Part model, mm, in its own coordinate system. A direction names the side the tool comes from. Coordinates: 2 decimals unless noted, no trailing zeros. Loops run counter-clockwise (first coordinate to the right, second up) from the corner with the lowest first, then second, coordinate; pieces in that order, holes last. Notation, with made-up numbers: (57.25, 63) -> (102.25, 63) arc R26 cw to (102.25, 92) -> close; hole circle Ø9 at (2, 33). An arc over 180 degrees is marked (long way). Use one line per item in the form item = value. Start each with the question number.
(1) Band-saw the part on D-D on y = 14.25. Give the cut face in (x, z), then the cut area to 3 significant figures.
(2) Band-saw the part on C-C on y = 8.5. Give the cut face in (x, z).
(3) Band-saw the part on B-B on x = 0. Give the cut face in (y, z), then the cut area to 3 significant figures.
(4) Drill centre lines: L1, parallel to Z at x = 0, y = 1.9; L2, parallel to Y at x = 0.5, z = -0.5; L3, parallel to Y at x = -2.75, z = -4.25. Where is each one in solid material? Low to high. Write a range as [from, to].
(5) Band-saw the part on A-A on z = 0. Give the cut face in (x, y), then the cut area to 3 significant figures.
(6) Pin check, flat tips, straight feed: P1, Ø1, axis at x = -2.5, y = 8, coming from the -Z side; P2, Ø1.5, axis at y = 3, z = 3.5, coming from the +X side; P3, Ø1.5, axis at x = 3.5, y = 10.5, coming from the -Z side. Stop position of each tip, or through.
(7) 3-axis set-ups, long thin cutter, end or side, ignore diameter. For faces 1 (the cylindrical face through (-5.39, 6.9, -1.7)), 2 (the flat face through (0, 3, 0)): which of +Z, -Z, +X, -X, +Y, -Y reach the whole face in a straight line?
Autodesk Inventor part; units mm, degrees
ref_plane "YZ Plane" through (0, 0, 0) normal (1, 0, 0) x (0, 1, 0)
ref_plane "XZ Plane" through (0, 0, 0) normal (0, 1, 0) x (-1, 0, 0)
ref_plane "XY Plane" through (0, 0, 0) normal (0, 0, 1) x (1, 0, 0)
sketch "Sketch1" plane through (0, 0, 0) normal (0, 1, 0) x (-1, 0, 0)
  circle A0 centre (0, 0) radius 5.65
  dimension "d0" = 11.3
extrude "Extrusion1" add sketch "Sketch1" along normal blind 15
sketch "Sketch2" plane through (0, 0, 0) normal (0, -1, 0) x (1, 0, 0)
  circle A0 centre (0, 0) radius 1.5
  dimension "d3" = 3
extrude "Extrusion2" cut sketch "Sketch2" against normal blind 3
fillet "Fillet1" radius 1 1 edges at (5.65, 15, 0)
properties part number "Pieza de Silicona"
A:
q1.outline = circle Ø11.24 at (0, 0)
q1.area = 99.2 mm²
q2.outline = circle Ø11.3 at (0, 0)
q3.outline = (0, -5.65) -> (14, -5.65) arc R1 ccw to (15, -4.65) -> (15, 4.65) arc R1 ccw to (14, 5.65) -> (0, 5.65) -> (0, 1.5) -> (3, 1.5) -> (3, -1.5) -> (0, -1.5) -> close
q3.area = 160 mm²
q4.L1 = [-5.65, -1.5], [1.5, 5.65]
q4.L2 = [3, 15]
q4.L3 = [0, 14.91]
q5.outline = (-5.65, 0) -> (-1.5, 0) -> (-1.5, 3) -> (1.5, 3) -> (1.5, 0) -> (5.65, 0) -> (5.65, 14) arc R1 ccw to (4.65, 15) -> (-4.65, 15) arc R1 ccw to (-5.65, 14) -> close
q5.area = 160 mm²
q6.P1 = -5.28
q6.P2 = 4.94
q6.P3 = -4.94
q7.face_1 = +Y, -Y
q7.face_2 = -Y
